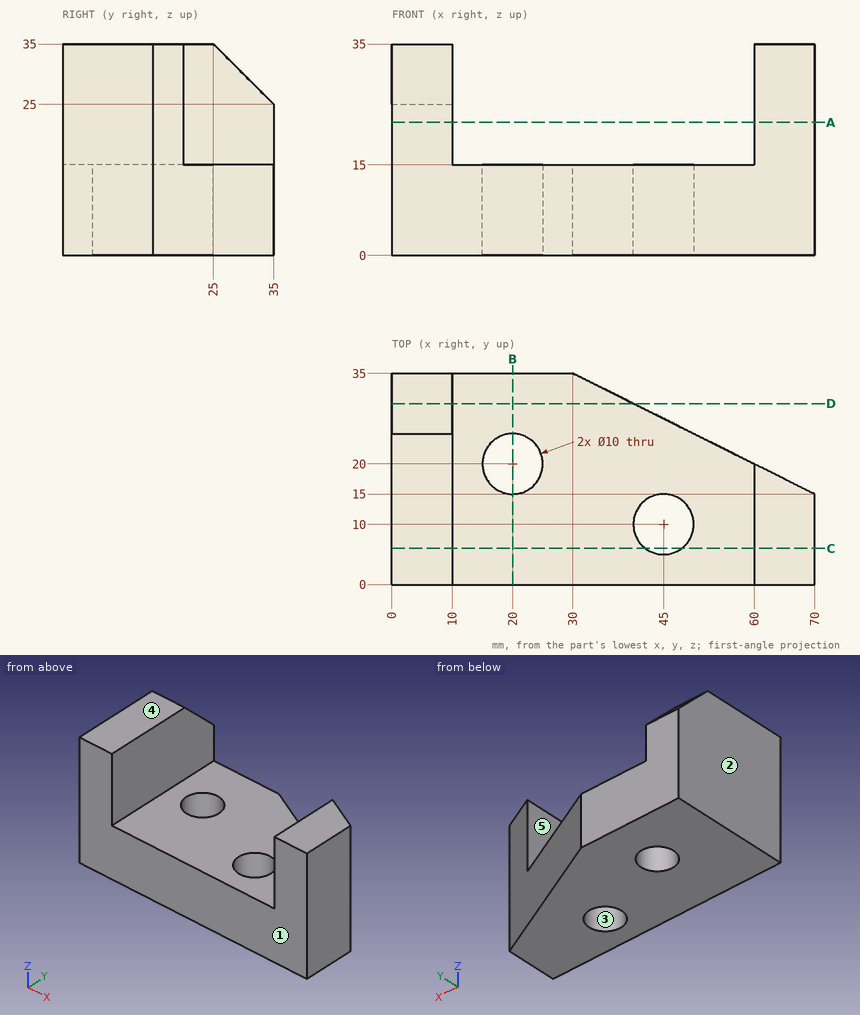
Job drawing, mm, ordinate dimensions from the low corner. One solid piece. A direction names the side the tool comes from. Give positions to 0.01 mm unless a question says otherwise; leave off trailing zeros. Write each loop counter-clockwise with the first axis right and the second up, starting at its lowest first coordinate (ties: lowest second). Pieces come first, ordered by that corner, then holes. Notation, with made-up numbers: (-34.5, 73) - (-29.5, 73) arc R14 cw to (-29.5, 95) - close; hole circle Ø5 at (-15, 69.5). An arc over 180 degrees is marked (long way). Answer as CSV lines item,"result".
1. Band-saw the part on C-C (y = 6). Write the cut outline in (x, z), and give its area (3 significant figures).
Responses:
outline,"(0, 0) - (42, 0) - (42, 15) - (10, 15) - (10, 35) - (0, 35) - close; (48, 0) - (70, 0) - (70, 35) - (60, 35) - (60, 15) - (48, 15) - close"
area,"1,360 mm2"
2. Drill centre lines: L1, parallel to X at y = 14, z = 30; L2, parallel to Y at x = 20, z = 7.25; L3, parallel to Z at x = 12, y = 29.5. Where is each one in solid material? Low to high. Write a range as [from, to].
Responses:
L1,"x = [0, 10], [60, 70]"
L2,"y = [0, 15], [25, 35]"
L3,"z = [0, 15]"
3. Pin check, flat tips, straight feed: pin 1 (2 mm diameter, centred on x = 34.5, y = 29, fed in from -Z); pin 2 (1 mm diameter, centred on y = 26.5, z = 20, fed in from +X); pin 3 (6 mm diameter, centred on x = 20, y = 20, fed in from +Z); pin 4 (13 mm diameter, centred on x = 45, y = 10, fed in from +Z). Stop position of each tip, or through.
Responses:
pin 1,"stops at z = 0"
pin 2,"stops at x = 10"
pin 3,"passes through"
pin 4,"stops at z = 15"
4. Band-saw the part on D-D (y = 30). Write the cut outline in (x, z).
Responses:
outline,"(0, 0) - (40, 0) - (40, 15) - (10, 15) - (10, 30) - (0, 30) - close"
5. Band-saw the part on B-B (x = 20). Write the cut outline in (y, z), and give its area (3 significant figures).
Responses:
outline,"(0, 0) - (15, 0) - (15, 15) - (0, 15) - close; (25, 0) - (35, 0) - (35, 15) - (25, 15) - close"
area,"375 mm2"
6. 3-axis set-ups, long thin cutter, end or side, ignore diameter. For the marked faces 4 and 5: which of +Z, -Z, +X, -X, +Y, -Y reach the whole face in a straight line?
Responses:
face 4,"+Z, +X, -X, +Y, -Y"
face 5,"+Z, +Y, -Y"
7. Two-plate mould, pull along Y, no slides. Class the marked faces 1, 2 and 3: +Y half, -Y half, draft (parallel to the pull), parting line (faces both ways), or undercut.
Responses:
face 1,"-Y half"
face 2,"draft"
face 3,"undercut"
8. Band-saw the part on A-A (z = 22). Write the cut outline in (x, y).
Responses:
outline,"(0, 0) - (10, 0) - (10, 35) - (0, 35) - close; (60, 0) - (70, 0) - (70, 15) - (60, 20) - close"
